Design review of the part built by this model. Coordinates are the model's own, in mm. Face numbers are marked on the shaded views. A direction names the side the tool comes from. Coordinates: 2 decimals unless noted, no trailing zeros. Order: outer loops, then holes, each group sorted by start corner. A loop starts at its lowest first (then second) coordinate and runs counter-clockwise, first axis right, second up. Notation, with made-up numbers: (63, 23.25) -> (109, 23.25) arc R21 cw to (109, 35.25) -> close; hole circle Ø8 at (16.25, 86). An arc over 180 degrees is marked (long way). Use a Markdown table: item, result. Add a question column.
Q1. Add section A-A (y = 0). State the section outline as (x, z) points (3 decimals).
Q2. Insertion check: pin 1 (1.5 mm diameter, centred on y = 8, z = -7, fed in from -X); pin 2 (5.5 mm diameter, centred on x = 0, y = 0, fed in from +Z); pin 3 (5 mm diameter, centred on y = -5.5, z = -11, fed in from +X); pin 4 (3 mm diameter, centred on y = -9.5, z = -11, fed in from +X). Each pin has a flat end and moves straight along its axis. Give the tip position at first contact, or say it passes through.
Q3. Machinability: for the marked faces 5, 6, 7 and 8, which of the approach directions +Z, -Z, +X, -X, +Y, -Y give a long, thin tool a straight path to every point of the face, cutting with its end or side? Answer none if there is none.
Q4. The part is to be moulded in two halves that separate along Z. For the marked faces 1, 2, 3 and 4, say which applies: pulls with the +Z half, pulls with the -Z half, needs draft (parallel to the pull), parting line crosses it, or undercut.
Q5. Add section D-D (y = 9.75). State the section outline as (x, z) points, then the cut area to 3 significant figures.
Q6. Wall thickness on probe 1 along Y at (x, z) = (0, -5.5) (3 decimals); probe 2 along Y at (x, z) = (0, -11.25) (3 decimals); probe 3 along Z at (x, y) = (-7, 6.5): over which ranges is each line inside the solid? List them lowest first.
Q7. Add section B-B (x = 0). State the section outline as (y, z) points (3 decimals), then the cut area to 3 significant figures.
Q8. Add section C-C (z = -12.5). State the section outline as (x, y) points (3 decimals), then the cut area to 3 significant figures.
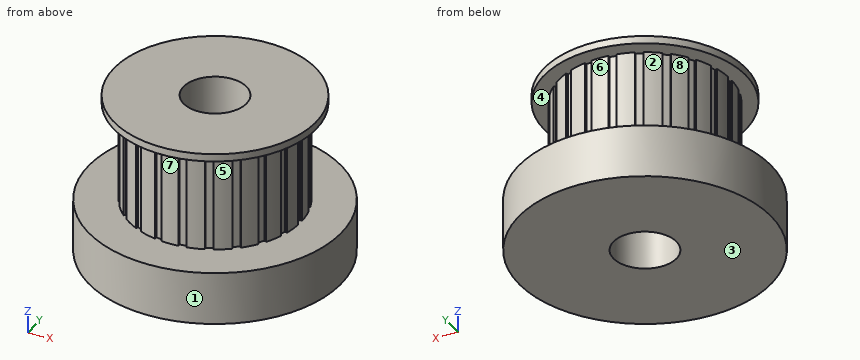
from build123d import *

# Parameters (mm, degrees)
SKETCH1_R           = 10.16
BOSS_EXTRUDE1_DEPTH = 0.762
SKETCH2_R           = 8.636
BOSS_EXTRUDE2_DEPTH = 10.16
SKETCH3_R           = 12.7
BOSS_EXTRUDE3_DEPTH = 5.334
SKETCH4_R           = 3.175
CUT_EXTRUDE1_DEPTH  = 25.654
SKETCH5_W           = 10.16
SKETCH5_H           = 0.762
CUT_EXTRUDE2_DEPTH  = 0.254
CIRPATTERN1_COUNT   = 22


with BuildPart() as part:
    # Sketch1 → Boss-Extrude1 (new body)
    with BuildSketch(Plane.XY):
        Circle(SKETCH1_R)
    extrude(amount=-BOSS_EXTRUDE1_DEPTH)

    # Sketch2 → Boss-Extrude2 (add)
    with BuildSketch(Plane(origin=(0, 0, -0.762), x_dir=(-1, 0, 0), z_dir=(0, 0, -1))):
        Circle(SKETCH2_R)
    extrude(amount=BOSS_EXTRUDE2_DEPTH)

    # Sketch3 → Boss-Extrude3 (add)
    with BuildSketch(Plane(origin=(0, 0, -10.922), x_dir=(-1, 0, 0), z_dir=(0, 0, -1))):
        Circle(SKETCH3_R)
    extrude(amount=BOSS_EXTRUDE3_DEPTH)

    # Sketch4 → Cut-Extrude1 (cut)
    with BuildSketch(Plane.XY):
        Circle(SKETCH4_R)
    extrude(amount=-CUT_EXTRUDE1_DEPTH, mode=Mode.SUBTRACT)

    # Sketch5 → Cut-Extrude2 (cut)
    with BuildSketch(Plane.ZY.offset(8.636)):
        with Locations((-5.842, 0)):
            Rectangle(SKETCH5_W, SKETCH5_H)
    cut_extrude2 = extrude(amount=-CUT_EXTRUDE2_DEPTH, mode=Mode.SUBTRACT)

    # CirPattern1: Cut-Extrude2 ×22 about axis
    cirpattern1_axis = Axis((0, 0, 0), (0, 0, 1))
    for i in range(1, CIRPATTERN1_COUNT):
        add(cut_extrude2.rotate(cirpattern1_axis, i * 360 / CIRPATTERN1_COUNT), mode=Mode.SUBTRACT)


solid = part.part
Established:
| question | item | result |
|---|---|---|
| 1 | outline | (-12.7, -16.256) -> (-3.175, -16.256) -> (-3.175, 0) -> (-10.16, 0) -> (-10.16, -0.762) -> (-8.382, -0.762) -> (-8.382, -10.922) -> (-12.7, -10.922) -> close; (3.175, -16.256) -> (12.7, -16.256) -> (12.7, -10.922) -> (8.382, -10.922) -> (8.382, -0.762) -> (10.16, -0.762) -> (10.16, 0) -> (3.175, 0) -> close |
| 2 | pin 1 | x = -4.69 |
| 2 | pin 2 | through |
| 2 | pin 3 | x = 12.34 |
| 2 | pin 4 | x = 9.86 |
| 3 | face 5 | +X, -Y |
| 3 | face 6 | +Y |
| 3 | face 7 | -Y |
| 3 | face 8 | -X, +Y |
| 4 | face 1 | needs draft |
| 4 | face 2 | undercut |
| 4 | face 3 | pulls with the -Z half |
| 4 | face 4 | undercut |
| 5 | outline | (-8.14, -16.26) -> (8.14, -16.26) -> (8.14, -10.92) -> (-8.14, -10.92) -> close; (-2.86, -0.76) -> (2.86, -0.76) -> (2.86, 0) -> (-2.86, 0) -> close |
| 5 | area | 91.2 mm^2 |
| 6 | probe 1 | -8.636 to -3.175, 3.175 to 8.636 |
| 6 | probe 2 | -12.7 to -3.175, 3.175 to 12.7 |
| 6 | probe 3 | -16.26 to -10.92, -0.76 to 0 |
| 7 | outline | (-12.7, -16.256) -> (-3.175, -16.256) -> (-3.175, 0) -> (-10.16, 0) -> (-10.16, -0.762) -> (-8.636, -0.762) -> (-8.636, -10.922) -> (-12.7, -10.922) -> close; (3.175, -16.256) -> (12.7, -16.256) -> (12.7, -10.922) -> (8.636, -10.922) -> (8.636, -0.762) -> (10.16, -0.762) -> (10.16, 0) -> (3.175, 0) -> close |
| 7 | area | 223 mm^2 |
| 8 | outline | circle Ø25.4 at (0, 0); hole circle Ø6.35 at (0, 0) |
| 8 | area | 475 mm^2 |
